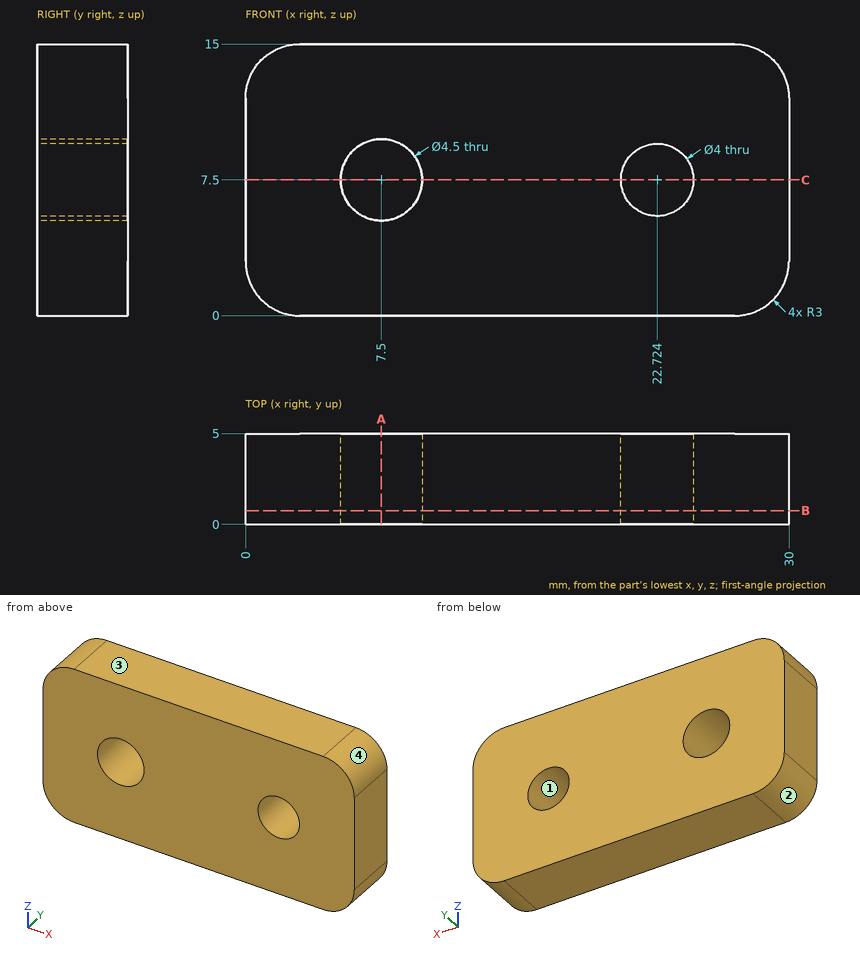
Could you check a few things on this drawing? It's one solid part, dimensions in mm from its lowest x, y, z. Give positions to 0.01 mm unless a question says otherwise; leave off trailing zeros. Order: outer loops, then holes, each group sorted by start corner. A loop starts at its lowest first (then second) coordinate and runs counter-clockwise, first axis right, second up. Notation, with made-up numbers: (21.25, 20) - (51.25, 20) arc R33 ccw to (51.25, 52) - close; hole circle Ø10 at (-31.5, 4.5). An arc over 180 degrees is marked (long way). Answer as a JSON object with one key per item and string values. Group by question number.
Item 1: If we section it at B-B on y = 0.75: Please give me the cut outline in (x, z), and give its area (3 significant figures).
Item 2: For P1, Ø3.5, axis at x = 7.5, z = 7.5, coming from the -Y side; P2, Ø3, axis at y = 3, z = 7.5, coming from the -X side, each with a flat end and sliding along its axis, tell me the tip position at first contact or that it passes through.
Item 3: Please list where these lines run through material, in increasing order: probe 1 along X at (y, z) = (2.75, 8) (1 decimal); probe 2 along Z at (x, y) = (7.5, 2.9); probe 3 along Z at (x, y) = (23, 3.8).
Item 4: If we mould it in two halves opening along X, with no side actions, what happens to the marked faces 1, 2, 3 and 4? For each: pulls with the +X half, pulls with the -X half, needs draft (parallel to the pull), parting line crosses it, or undercut.
Item 5: If we section it at C-C on z = 7.5: Please give me the cut outline in (x, y).
Item 6: If we section it at A-A on x = 7.5: Please give me the cut outline in (y, z), and give its area (3 significant figures).
Result set:
{
 "1": {"outline": "(0, 3) arc R3 ccw to (3, 0) - (27, 0) arc R3 ccw to (30, 3) - (30, 12) arc R3 ccw to (27, 15) - (3, 15) arc R3 ccw to (0, 12) - close; hole circle Ø4.5 at (7.5, 7.5); hole circle Ø4 at (22.72, 7.5)", "area": "414 mm²"},
 "2": {"P1": "through", "P2": "x = 0"},
 "3": {"probe 1": "0 to 5.3, 9.7 to 20.8, 24.7 to 30", "probe 2": "0 to 5.25, 9.75 to 15", "probe 3": "0 to 5.52, 9.48 to 15"},
 "4": {"face 1": "undercut", "face 2": "pulls with the -X half", "face 3": "needs draft", "face 4": "pulls with the +X half"},
 "5": {"outline": "(0, 0) - (5.25, 0) - (5.25, 5) - (0, 5) - close; (9.75, 0) - (20.72, 0) - (20.72, 5) - (9.75, 5) - close; (24.72, 0) - (30, 0) - (30, 5) - (24.72, 5) - close"},
 "6": {"outline": "(0, 0) - (5, 0) - (5, 5.25) - (0, 5.25) - close; (0, 9.75) - (5, 9.75) - (5, 15) - (0, 15) - close", "area": "52.5 mm²"}
}
